Source: CAD feature listing. Evaluate the final solid. Frame: model axes, mm. A direction names the side the tool comes from. Coordinates: 2 decimals unless noted, no trailing zeros. Order: outer loops, then holes, each group sorted by start corner. A loop starts at its lowest first (then second) coordinate and runs counter-clockwise, first axis right, second up.
```python
from build123d import *

# Parameters (mm, degrees)
FILLET_R     = 5
POCKET_DEPTH = 5
FILLET003_R  = 2


with BuildPart() as part:
    # Sketch001 → Revolution001 (revolve)
    with BuildSketch(Plane.XY):
        Polygon((0, 0), (-72, 0), (-72, -25), (-75, -25), (-75, 0), (-75, 2), (0, 2), align=None)
    revolve(axis=Axis((0, 0, 0), (0, 1, 0)))

    # Fillet
    fillet_edges = [part.edges().sort_by_distance(p)[0] for p in [
        (72, 0, 0),
    ]]
    fillet(fillet_edges, radius=FILLET_R)

    # Sketch002 (on Face1 of Fillet) → Pocket (cut)
    with BuildSketch(Plane.XZ):
        with BuildLine():
            ThreePointArc((-65, 2), (-67, 0), (-65, -2))
            Line((-65, -2), (65, -2))
            ThreePointArc((65, -2), (67, 0), (65, 2))
            Line((-65, 2), (65, 2))
        make_face()
        with BuildLine():
            ThreePointArc((-64.505814, 10), (-66.505814, 8), (-64.505814, 6))
            Line((-64.505814, 6), (64.505814, 6))
            ThreePointArc((64.505814, 6), (66.505814, 8), (64.505814, 10))
            Line((-64.505814, 10), (64.505814, 10))
        make_face()
        with BuildLine():
            ThreePointArc((-63, 18), (-65, 16), (-63, 14))
            Line((-63, 14), (63, 14))
            ThreePointArc((63, 14), (65, 16), (63, 18))
            Line((-63, 18), (63, 18))
        make_face()
        with BuildLine():
            ThreePointArc((-60.406953, 26), (-62.406953, 24), (-60.406953, 22))
            Line((-60.406953, 22), (60.406953, 22))
            ThreePointArc((60.406953, 22), (62.406953, 24), (60.406953, 26))
            Line((-60.406953, 26), (60.406953, 26))
        make_face()
        with BuildLine():
            ThreePointArc((-56.577381, 34), (-58.577381, 32), (-56.577381, 30))
            Line((-56.577381, 30), (56.577381, 30))
            ThreePointArc((56.577381, 30), (58.577381, 32), (56.577381, 34))
            Line((-56.577381, 34), (56.577381, 34))
        make_face()
        with BuildLine():
            ThreePointArc((-51.234754, 42), (-53.234754, 40), (-51.234754, 38))
            Line((-51.234754, 38), (51.234754, 38))
            ThreePointArc((51.234754, 38), (53.234754, 40), (51.234754, 42))
            Line((-51.234754, 42), (51.234754, 42))
        make_face()
        with BuildLine():
            ThreePointArc((-43.829214, 50), (-45.829214, 48), (-43.829214, 46))
            Line((-43.829214, 46), (43.829214, 46))
            ThreePointArc((43.829214, 46), (45.829214, 48), (43.829214, 50))
            Line((-43.829214, 50), (43.829214, 50))
        make_face()
        with BuildLine():
            ThreePointArc((-33, 58), (-35, 56), (-33, 54))
            Line((-33, 54), (33, 54))
            ThreePointArc((33, 54), (35, 56), (33, 58))
            Line((-33, 58), (33, 58))
        make_face()
        with BuildLine():
            ThreePointArc((-64.505814, -6), (-66.505814, -8), (-64.505814, -10))
            Line((-64.505814, -10), (64.505814, -10))
            ThreePointArc((64.505814, -10), (66.505814, -8), (64.505814, -6))
            Line((-64.505814, -6), (64.505814, -6))
        make_face()
        with BuildLine():
            ThreePointArc((-63, -14), (-65, -16), (-63, -18))
            Line((-63, -18), (63, -18))
            ThreePointArc((63, -18), (65, -16), (63, -14))
            Line((-63, -14), (63, -14))
        make_face()
        with BuildLine():
            ThreePointArc((-60.406953, -22), (-62.406953, -24), (-60.406953, -26))
            Line((-60.406953, -26), (60.406953, -26))
            ThreePointArc((60.406953, -26), (62.406953, -24), (60.406953, -22))
            Line((-60.406953, -22), (60.406953, -22))
        make_face()
        with BuildLine():
            ThreePointArc((-56.577381, -30), (-58.577381, -32), (-56.577381, -34))
            Line((-56.577381, -34), (56.577381, -34))
            ThreePointArc((56.577381, -34), (58.577381, -32), (56.577381, -30))
            Line((-56.577381, -30), (56.577381, -30))
        make_face()
        with BuildLine():
            ThreePointArc((-51.234754, -38), (-53.234754, -40), (-51.234754, -42))
            Line((-51.234754, -42), (51.234754, -42))
            ThreePointArc((51.234754, -42), (53.234754, -40), (51.234754, -38))
            Line((-51.234754, -38), (51.234754, -38))
        make_face()
        with BuildLine():
            ThreePointArc((-43.829214, -46), (-45.829214, -48), (-43.829214, -50))
            Line((-43.829214, -50), (43.829214, -50))
            ThreePointArc((43.829214, -50), (45.829214, -48), (43.829214, -46))
            Line((-43.829214, -46), (43.829214, -46))
        make_face()
        with BuildLine():
            ThreePointArc((-33, -54), (-35, -56), (-33, -58))
            Line((-33, -58), (33, -58))
            ThreePointArc((33, -58), (35, -56), (33, -54))
            Line((-33, -54), (33, -54))
        make_face()
    extrude(amount=-POCKET_DEPTH, mode=Mode.SUBTRACT)

    # Fillet003
    fillet003_edges = [part.edges().sort_by_distance(p)[0] for p in [
        (75, -25, 0),
    ]]
    fillet(fillet003_edges, radius=FILLET003_R)


solid = part.part
```
1. Access query for faces 5 (the face through (0, 0, 61)), 6 (the face through (1, 2, 34.4)). Directions: +Z, -Z, +X, -X, +Y, -Y. A direction counts if a zero-diameter tool reaches every point of the face in a straight line with its end or side. Return the directions, or none.
Findings:
face 5: -Y
face 6: +Z, -Z, +X, -X, +Y
2. Pin query (flat end, axial travel): P1, Ø1, axis at x = 17, y = 1.5, coming from the +Z side; P2, Ø1.6, axis at x = 14.5, y = 1, coming from the -Z side; P3, Ø8, axis at x = 39.5, y = -14, coming from the +Z side. Return the tip coordinate at first contact, or that it passes through.
Findings:
P1: stops at z = 73.16
P2: stops at z = -73.74
P3: stops at z = 66.07
3. Section query A-A on y = -14.5. Return loops of the section in (x, z), plus the area to 3 significant figures.
Findings:
outline: circle Ø150 at (0, 0); hole circle Ø144 at (0, 0)
area: 1,390 mm2
4. Section query B-B on x = 16. Count the separate pieces of the cut face and the enclosed holes in it, plus the area to 3 significant figures.
Findings:
separate pieces: 16
enclosed holes: 0
area: 336 mm2
5. Ray query, line 1 (Z direction, x = 0, y = -19.75); line 2 (Z direction, x = 66, y = 0.75); line 3 (Y direction, x = 28, z = 35). Return the intervals inside material, ascending.
Findings:
line 1: z = -75 to -72, 72 to 75
line 2: z = -35.62 to -9.33, -6.67 to -1.73, 1.73 to 6.67, 9.33 to 35.62
line 3: y = 0 to 2
6. Draft query along Z for faces 1 (the face through (-1, 0, 52)), 2 (the face through (54, -25, -48)), 3 (the face through (9.764, -10.675, 74.362)), 4 (the face through (-1, 0, 12)). Return one class per face: released by +Z, released by -Z, zero draft, split by the parting line, or undercut.
Findings:
face 1: undercut
face 2: zero draft
face 3: split by the parting line
face 4: undercut
